Autodesk Fusion 360 part; units mm, degrees
sketch "Esquisse1" plane through (0, 0, 0) normal (0, 0, 1) x (1, 0, 0)
  line L0 (0, 0) -> (53.34, 0)
  line L1 (53.34, 0) -> (53.34, 66.04)
  line L2 (48.06, 68.58) -> (15.49, 68.58)
  line L3 (0, 66.04) -> (0, 0)
  line L4 (12.95, 66.04) -> (0, 66.04)
  line L5 (12.95, 66.04) -> (15.49, 68.58)
  line L6 (12.95, 66.04) -> (16.5421, 66.04) construction
  line L7 (50.6, 66.04) -> (53.34, 66.04)
  line L8 (50.6, 66.04) -> (48.06, 68.58)
  line L9 (50.6, 66.04) -> (54.1921, 66.04) construction
  line L10 (0, 0) -> (2.54, 0)
  line L11 (0, 15.24) -> (0, 0)
  line L12 (53.34, 0) -> (50.8, 0)
  line L13 (53.34, 13.97) -> (53.34, 0)
  line L14 (53.34, 66.04) -> (50.6, 66.04)
  line L15 (0, 66.04) -> (12.95, 66.04)
  line L16 (-0.3, 66.04) -> (-0.3, 56.04)
  line L17 (0, 56.04) -> (0, 66.04)
  line L18 (0, 66.04) -> (10, 66.04)
  line L19 (10, 66.34) -> (-0.3, 66.34)
  line L20 (-0.3, 66.34) -> (-0.3, 66.04)
  line L21 (-0.3, 56.04) -> (-3.3, 56.04)
  line L22 (-3.3, 56.04) -> (-3.3, 66.34)
  line L23 (-0.3, 66.34) -> (-0.3, 56.04)
  line L24 (10, 66.34) -> (-0.3, 66.34)
  line L25 (-0.3, 69.34) -> (10, 69.34)
  line L26 (10, 69.34) -> (10, 66.34)
  line L27 (-3.3, 66.34) -> (-3.3, 69.34)
  line L28 (-3.3, 69.34) -> (-0.3, 69.34)
  line L29 (-0.2984, 0.0305) -> (-0.2984, 9.0305)
  line L30 (0, 9) -> (0, 0)
  line L31 (0, 0) -> (9.0015, 0)
  line L32 (9.0015, -0.2695) -> (-0.2984, -0.2695)
  line L33 (-0.2984, -0.2695) -> (-0.2984, 0.0305)
  line L34 (-0.2984, 9.0305) -> (-3.2984, 9.0305)
  line L35 (-3.2984, 9.0305) -> (-3.2984, -0.3)
  line L36 (-0.2984, -0.2695) -> (-0.2984, 9.0305)
  line L37 (9.0015, -0.2695) -> (0.0015, -0.2695)
  line L38 (0, 0) -> (0, 2.7305)
  line L39 (9.0015, -0.2695) -> (-0.2984, -0.2695)
  line L40 (-3.2984, -0.3) -> (-3.2984, -3.2695)
  line L41 (-3.2984, -3.2695) -> (9.0015, -3.2695)
  line L42 (9.0015, -3.2695) -> (9.0015, -0.2695)
  line L43 (53.34, 0) -> (53.34, 33.02)
  line L44 (53.64, 33.02) -> (53.64, 43.02)
  line L45 (53.34, 43.02) -> (53.34, 33.02)
  line L46 (53.64, 33.02) -> (53.64, 23.02)
  line L47 (53.64, 43.02) -> (56.64, 43.02)
  line L48 (56.64, 43.02) -> (56.64, 23.02)
  line L49 (56.64, 23.02) -> (53.64, 23.02)
  line L50 (53.64, 23.02) -> (53.64, 43.02)
  circle A0 centre (45.72, 66.04) radius 1.5
  circle A1 centre (17.78, 66.04) radius 1.5
  circle A2 centre (50.8, 13.97) radius 1.5
  circle A3 centre (2.54, 15.24) radius 1.5
  line L51 (-3.2985, -8.2695) -> (-8.2985, -8.2695)
  line L52 (56.64, 74.34) -> (61.64, 74.34)
  line L53 (-8.2985, -8.2695) -> (61.64, -8.2695)
  line L54 (61.64, -8.2695) -> (61.64, 74.34)
  line L55 (61.64, 74.34) -> (-8.2985, 74.34)
  line L56 (-8.2985, 74.34) -> (-8.2985, -8.2695)
  line L57 (-8.2985, 74.34) -> (-8.2985, 71.34)
  line L58 (-5.2985, 71.34) -> (58.64, 71.34)
  line L59 (-8.2985, -8.2695) -> (-5.2985, -8.2695)
  line L60 (-8.2985, -5.2695) -> (-8.2985, -8.2695)
  line L61 (-5.2985, -5.2695) -> (-5.2985, 71.34)
  line L62 (61.64, -8.2695) -> (58.64, -8.2695)
  line L63 (61.64, -5.2695) -> (61.64, -8.2695)
  line L64 (61.64, 74.34) -> (58.64, 74.34)
  line L65 (61.64, 71.34) -> (61.64, 74.34)
  line L66 (58.64, 71.34) -> (58.64, -5.2695)
  line L67 (-5.2985, -5.2695) -> (58.64, -5.2695)
  line L68 (61.64, 74.34) -> (60.14, 74.34)
  line L69 (60.14, 74.34) -> (60.14, 72.84)
  line L70 (60.14, 72.84) -> (61.64, 72.84)
  line L71 (61.64, 72.84) -> (61.64, 74.34)
  circle A4 centre (60.14, 72.84) radius 3
  line L72 (61.64, -8.2695) -> (60.14, -8.2695)
  line L73 (60.14, -8.2695) -> (60.14, -6.7695)
  line L74 (60.14, -6.7695) -> (61.64, -6.7695)
  line L75 (61.64, -6.7695) -> (61.64, -8.2695)
  circle A5 centre (60.14, -6.7695) radius 3
  line L76 (-8.2985, -8.2695) -> (-6.7985, -8.2695)
  line L77 (-6.7985, -8.2695) -> (-6.7985, -6.7695)
  line L78 (-6.7985, -6.7695) -> (-8.2985, -6.7695)
  line L79 (-8.2985, -6.7695) -> (-8.2985, -8.2695)
  circle A6 centre (-6.7985, -6.7695) radius 3
  line L80 (-8.2985, 74.34) -> (-6.7985, 74.34)
  line L81 (-6.7985, 74.34) -> (-6.7985, 72.84)
  line L82 (-6.7985, 72.84) -> (-8.2985, 72.84)
  line L83 (-8.2985, 72.84) -> (-8.2985, 74.34)
  circle A7 centre (-6.7985, 72.84) radius 3
  dimension "LargeurArduino" = 53.34
  dimension "d5" = 45
  dimension "d8" = 135
  dimension "d9" = 17.78
  dimension "d10" = 7.62
  dimension "d13" = 2.54
  dimension "d14" = 15.24
  dimension "d15" = 2.54
  dimension "d16" = 13.97
  dimension "DistanceMorsArduino" = 0.3
  dimension "d27" = 10
  dimension "d28" = 10.3
  dimension "d29" = 0.3
  dimension "d30" = 3
  dimension "d31" = 10.3
  dimension "d32" = 10.3
  dimension "d33" = 3
  dimension "d34" = 3
  dimension "d35" = 3
  dimension "d36" = 0.3
  dimension "d37" = 9
  dimension "d38" = 9.3
  dimension "d39" = 0.3
  dimension "d40" = 3
  dimension "d41" = 9.3
  dimension "d42" = 9
  dimension "d44" = 12.3
  dimension "d45" = 3
  dimension "d46" = 33.02
  dimension "d47" = 0.3
  dimension "d48" = 10
  dimension "d49" = 0.3
  dimension "d51" = 3
  dimension "d52" = 20
  dimension "d54" = 3
  dimension "d55" = 3
  dimension "d56" = 3
  dimension "d59" = 5
  dimension "d60" = 5
  dimension "d63" = 5
  dimension "EpaisseurBoitier" = 3
  dimension "d65" = 3
  dimension "d66" = 3
  dimension "d67" = 3
  dimension "d68" = 3
  dimension "d69" = 3
  dimension "d70" = 3
  dimension "d71" = 3
  dimension "d72" = 1.5
  dimension "d73" = 1.5
  dimension "d74" = 6
  dimension "d75" = 1.5
  dimension "d76" = 1.5
  dimension "d77" = 6
  dimension "d78" = 1.5
  dimension "d79" = 1.5
  dimension "d80" = 6
  dimension "d81" = 1.5
  dimension "d82" = 1.5
  dimension "d83" = 6
sketch "Esquisse10" plane through (0, 0, 0) normal (0, 0, 1) x (1, 0, 0)
sketch "Esquisse9" plane through (0, 0, 0) normal (0, 0, 1) x (1, 0, 0)
sketch "Esquisse2" plane through (0, 0, 0) normal (0, 0, 1) x (1, 0, 0)
sketch "Esquisse13" plane through (0, 0, 0) normal (0, 0, 1) x (1, 0, 0)
sketch "Esquisse11" plane through (0, 0, 0) normal (0, 0, 1) x (1, 0, 0)
  line L0 (0, 66) -> (1, 66)
  line L1 (1, 66) -> (4, 66)
  line L2 (4, 66) -> (4, 17)
  line L3 (4, 17) -> (1, 17)
  line L4 (1, 17) -> (1, 66)
  line L5 (53, 66) -> (52, 66)
  line L6 (52, 66) -> (49, 66)
  line L7 (49, 66) -> (49, 26)
  line L8 (49, 26) -> (52, 26)
  line L9 (52, 26) -> (52, 66)
  line L10 (0, 0) -> (5, 0)
  line L11 (5, 0) -> (5, 8)
  line L12 (5, 8) -> (0, 8)
  line L13 (0, 8) -> (0, 0)
  circle A0 centre (5, 8) radius 4
  dimension "d157" = 1
  dimension "d158" = 3
  dimension "d159" = 49
  dimension "d160" = 1
  dimension "d161" = 3
  dimension "d162" = 40
  dimension "d163" = 5
  dimension "d164" = 8
  dimension "d165" = 8
extrude "Extrusion15" add sketch "Esquisse11" sketch "Esquisse1" along normal blind 3 of sketch 2 contours L0 L1 L2 L3 L4 L5 L7 L8 L10 L11 L12 L13 L14 L15 L17 L18 L30 L31 L38 L43 L45 | L16 L19 L20 L21 L22 L23 L24 L25 L26 L27 L28 | L29 L32 L33 L34 L35 L36 L37 L39 L40 L41 L42 | L44 L46 L47 L48 L49 L50 | A0 | A1 | A2 | A3 | L51 L53 L56 L59 L60 L76 L79 A6 | L51 L53 L56 L59 L60 L61 L67 L77 L78 A6 | L51 L53 L56 L59 L60 L76 L77 L78 L79 | L51 L53 L67 A5 A6 | L56 L61 A6 A7 | L53 L54 L62 L63 L66 L67 L73 L74 A5 | L53 L54 L62 L63 L72 L75 A5 | L55 L56 L57 L80 L83 A7 | L55 L56 L57 L58 L61 L81 L82 A7 | L61 L67 A6 | L58 L61 L66 L67 A4 A5 A6 A7 | L66 L67 A5 | L52 L55 L58 A4 A7 | L58 L61 A7 | L53 L54 L62 L63 L72 L73 L74 L75 | L54 L66 A4 A5 | L55 L56 L57 L80 L81 L82 L83 | L58 L66 A4 | L52 L54 L55 L58 L64 L65 L66 L69 L70 A4 | L52 L54 L55 L64 L65 L68 L71 A4 | L52 L54 L55 L64 L65 L68 L69 L70 L71
sketch "Esquisse12" plane through (0, 0, 0) normal (0, 0, 1) x (1, 0, 0)
sketch "Esquisse14" plane through (0, 0, 0) normal (0, 0, 1) x (1, 0, 0)
extrude "Extrusion16" cut sketch "Esquisse11" along normal blind 15 contours L11 L12 A0 | L11 L12 A0
extrude "Extrusion17" cut sketch "Esquisse11" along normal blind 5 contours L6 L7 L8 L9
extrude "Extrusion18" cut sketch "Esquisse11" along normal blind 5 contours L1 L2 L3 L4
sketch "Esquisse15" plane through (0, 0, 0) normal (0, 0, 1) x (1, 0, 0)
  circle A0 centre (-6.7985, 72.84) radius 1.5
  circle A1 centre (60.14, 72.84) radius 1.5
  circle A2 centre (-6.7985, -6.7695) radius 1.5
  circle A3 centre (60.14, -6.7695) radius 1.5
  point P0 (-6.7985, 72.84)
  point P1 (60.14, 72.84)
  point P2 (-6.7985, 72.84)
  point P3 (-6.7985, -6.7695)
  point P4 (60.14, -6.7695)
  dimension "d174" = 3
  dimension "d175" = 3
  dimension "d176" = 3
  dimension "d177" = 3
extrude "Extrusion19" cut sketch "Esquisse15" along normal blind 3
sketch "Esquisse16" plane through (0, 0, 3) normal (0, 0, 1) x (-1, 0, 0)
  circle A0 centre (-60.14, -72.84) radius 1.5
  circle A1 centre (6.7985, 6.7695) radius 1.5
  circle A2 centre (6.7985, -72.84) radius 1.5
  circle A3 centre (-60.14, 6.7695) radius 1.5
  line L0 (-1, -17) -> (-1, -66)
  line L1 (-1, -66) -> (-4, -66)
  line L2 (-4, -66) -> (-4, -17)
  line L3 (-4, -17) -> (-1, -17)
  line L4 (-52, -26) -> (-49, -26)
  line L5 (-49, -26) -> (-49, -66)
  line L6 (-49, -66) -> (-52, -66)
  line L7 (-52, -66) -> (-52, -26)
  circle A4 centre (-5, -8) radius 4
  line L8 (-57.5419, -74.34) -> (4.2004, -74.34)
  arc A5 (4.2004, -74.34) -> (8.2985, -70.2419) centre (6.7985, -72.84) ccw
  line L9 (8.2985, -70.2419) -> (8.2985, 4.1714)
  arc A6 (8.2985, 4.1714) -> (4.2004, 8.2695) centre (6.7985, 6.7695) ccw
  line L10 (4.2004, 8.2695) -> (-57.5419, 8.2695)
  arc A7 (-57.5419, 8.2695) -> (-61.64, 4.1714) centre (-60.14, 6.7695) ccw
  line L11 (-61.64, 4.1714) -> (-61.64, -70.2419)
  arc A8 (-61.64, -70.2419) -> (-57.5419, -74.34) centre (-60.14, -72.84) ccw
  line L12 (-39.0942, -3.1233) -> (-39.3144, -74.255) construction
  line L13 (-39.3144, -74.255) -> (-11.8714, -74.34) construction
  line L14 (-11.8714, -74.34) -> (-11.6511, -3.2083) construction
  line L15 (-11.6511, -3.2083) -> (-39.0942, -3.1233) construction
  dimension "d180" = 10
component "CouvercleArduino" placed x (1, 0, 0) y (0, 1, 0) z (0, 0, 1) at (0, 0, 0)
equation "d29 = DistanceMorsArduino"
equation "d30 = EpaisseurMors"
equation "d33 = EpaisseurMors"
equation "d36 = DistanceMorsArduino"
equation "d39 = DistanceMorsArduino"
equation "d40 = EpaisseurMors"
equation "d45 = EpaisseurMors"
equation "d47 = DistanceMorsArduino"
equation "d49 = DistanceMorsArduino"
equation "d51 = EpaisseurMors"
equation "d54 = Diameter Dimension-7"
equation "d55 = Diameter Dimension-8"
equation "d56 = Diameter Dimension-9"
equation "d59 = DistanceMorsBoitier"
equation "d60 = DistanceMorsBoitier"
equation "d63 = DistanceMorsBoitier"
equation "d65 = EpaisseurBoitier"
equation "d66 = EpaisseurBoitier"
equation "d67 = EpaisseurBoitier"
equation "d68 = EpaisseurBoitier"
equation "d69 = EpaisseurBoitier"
equation "d70 = EpaisseurBoitier"
equation "d71 = EpaisseurBoitier"
equation "d72 = EpaisseurBoitier / 2"
equation "d73 = EpaisseurBoitier / 2"
equation "d74 = EpaisseurBoitier * 2"
equation "d75 = EpaisseurBoitier / 2"
equation "d76 = EpaisseurBoitier / 2"
equation "d77 = EpaisseurBoitier * 2"
equation "d78 = EpaisseurBoitier / 2"
equation "d79 = EpaisseurBoitier / 2"
equation "d80 = EpaisseurBoitier * 2"
equation "d81 = EpaisseurBoitier / 2"
equation "d82 = EpaisseurBoitier / 2"
equation "d83 = EpaisseurBoitier * 2"
equation "HauteurMors = 5 mm"
equation "HauteurBoitier = 25 mm"
equation "mm = 1 mm"
equation "d174 = Diameter Dimension-2"
equation "d175 = Diameter Dimension-3"
equation "d176 = Diameter Dimension-4"
equation "d177 = Diameter Dimension-5"
Work out the finished part from the listing and answer in its coordinate system (mm). A direction names the side the tool comes from. Give positions to 0.01 mm unless a question says otherwise; leave off trailing zeros. Loops run counter-clockwise (first coordinate to the right, second up) from the corner with the lowest first, then second, coordinate; pieces in that order, holes last. Notation, with made-up numbers: (66.25, 74) -> (125.25, 74) arc R26 cw to (125.25, 90) -> close; hole circle Ø2 at (27.5, 9.5). An arc over 180 degrees is marked (long way). One line per question, with ' | ' between items. Start each with the question number.
1) Section A-A, the plane x = 51 is taken. Determine the outline of the cut face in (y, z).
2) Section B-B, the plane y = 8 is taken. Determine the outline of the cut face in (x, z), then the cut area to 3 significant figures.
3) Section C-C, the plane x = 60.14 is taken. Determine the outline of the cut face in (y, z).
4) Straight lines are drawn through the part: L1, parallel to X at y = 31, z = 2.25; L2, parallel to X at y = 8, z = 1.8; L3, parallel to X at y = 21, z = 1.1. For each, find the intervals that lie inside material, in ascending order.
5) Each of these flat-tipped pins is pushed along its axis until it touches: pin 1 (1.5 mm diameter, centred on y = 32.5, z = 1.5, fed in from -X); pin 2 (3.5 mm diameter, centred on x = -6.8, y = 72.84, fed in from +Z); pin 3 (1.5 mm diameter, centred on y = 19, z = 1, fed in from +X); pin 4 (1.5 mm diameter, centred on x = 2, z = 2, fed in from +Y). Where does it stop, or does it pass through?
6) Section D-D, the plane y = 60 is taken. Determine the outline of the cut face in (x, z).
7) Determine the mould class of faces 1 (the face through (26, -8.27, 1)), 2 (the face through (3, 17, 1)), 3 (the face through (26, 34, 3)) for opening direction Y: +Y half, -Y half, draft (parallel to the pull), parting line (faces both ways), or undercut.
8) For faces 4 (the face through (51, 66, 1)), 5 (the face through (61.64, 33, 1)), 6 (the face through (27, 74.34, 1)), determine the directions among +Z, -Z, +X, -X, +Y, -Y from which every point of the face is accessible in a straight line to the end or side of a thin tool.
Resolved:
1) outline: (-8.27, 0) -> (26, 0) -> (26, 3) -> (-8.27, 3) -> close; (66, 0) -> (74.34, 0) -> (74.34, 3) -> (66, 3) -> close
2) outline: (-8.3, 0) -> (1, 0) -> (1, 3) -> (-8.3, 3) -> close; (9, 0) -> (61.64, 0) -> (61.64, 3) -> (9, 3) -> close | area: 186 mm2
3) outline: (-9.77, 0) -> (-8.27, 0) -> (-8.27, 3) -> (-9.77, 3) -> close; (-5.27, 0) -> (71.34, 0) -> (71.34, 3) -> (-5.27, 3) -> close; (74.34, 0) -> (75.84, 0) -> (75.84, 3) -> (74.34, 3) -> close
4) L1: -8.3 to 1, 4 to 49, 52 to 61.64 | L2: -8.3 to 1, 9 to 61.64 | L3: -8.3 to 1, 4 to 61.64
5) pin 1: x = -8.3 | pin 2: z = 3 | pin 3: x = 61.64 | pin 4: y = 74.34
6) outline: (-8.3, 0) -> (1, 0) -> (1, 3) -> (-8.3, 3) -> close; (4, 0) -> (49, 0) -> (49, 3) -> (4, 3) -> close; (52, 0) -> (61.64, 0) -> (61.64, 3) -> (52, 3) -> close
7) face 1: -Y half | face 2: undercut | face 3: draft
8) face 4: +Z, -Z | face 5: +Z, -Z, +X | face 6: +Z, -Z, +Y
